CAD build for the part. Positions are in the model's coordinates, mm. Round coordinates to 2 decimals unless told otherwise and drop trailing zeros. Order: outer loops, then holes, each group sorted by start corner. A loop starts at its lowest first (then second) coordinate and runs counter-clockwise, first axis right, second up. Notation, with made-up numbers: (-16.75, -9) - (15.25, -9) arc R5 ccw to (15.25, -3) - close; hole circle Ø9 at (-27.5, 27.25). An arc over 180 degrees is marked (long way). Use one line per item in the form item = value. Start each with the question number.
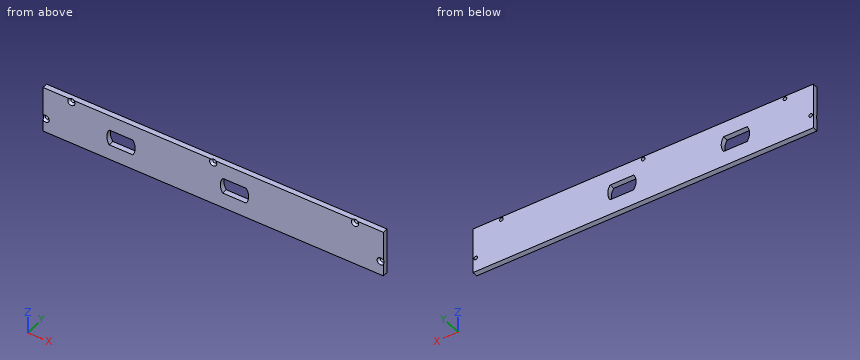
from build123d import *

# Parameters (mm, degrees)
F0_W           = 304.8
F0_H           = 41.275
F1_DEPTH       = 4.7625
F3_D           = 3.2639
F3_DEPTH       = 14.605
F3_CSINK_D     = 6.477
F3_CSINK_ANGLE = 82
F3_TIP         = 0.9805744872
F5_DEPTH       = 25.4


with BuildPart() as f1:
    # F0 (on Front) → F1 (new body)
    with BuildSketch(Plane.XZ):
        with Locations((33.2768968371, 36.1280379981)):
            Rectangle(F0_W, F0_H)
    extrude(amount=F1_DEPTH)

    # F3
    with Locations(Plane.XZ.offset(4.7625)):
        with Locations((-93.7231031629, 54.3842879981), (-116.7418531629, 28.1905379981), (33.2768968371, 54.3842879981), (160.2768968371, 54.3842879981), (183.2956468371, 28.1905379981)):
            CounterSinkHole(F3_D / 2, F3_CSINK_D / 2, depth=F3_DEPTH, counter_sink_angle=F3_CSINK_ANGLE)
            with Locations((0, 0, -(F3_DEPTH + F3_TIP / 2))):  # 118° drill point
                Cone(0, F3_D / 2, F3_TIP, mode=Mode.SUBTRACT)

    # F4 (on face) → F5 (cut)
    with BuildSketch(Plane.XZ.offset(4.7625)):
        with BuildLine():
            Line((-38.6665120517, 43.1130379981), (-59.879694274, 43.1130379981))
            ThreePointArc((-59.879694274, 43.1130379981), (-61.9731031629, 36.1280379981), (-59.879694274, 29.1430379981))
            Line((-59.879694274, 29.1430379981), (-38.6665120517, 29.1430379981))
            ThreePointArc((-38.6665120517, 29.1430379981), (-36.5731031629, 36.1280379981), (-38.6665120517, 43.1130379981))
        make_face()
        with BuildLine():
            ThreePointArc((62.9334879483, 29.1430379981), (65.0268968371, 36.1280379981), (62.9334879483, 43.1130379981))
            Line((62.9334879483, 43.1130379981), (41.720305726, 43.1130379981))
            ThreePointArc((41.720305726, 43.1130379981), (39.6268968371, 36.1280379981), (41.720305726, 29.1430379981))
            Line((41.720305726, 29.1430379981), (62.9334879483, 29.1430379981))
        make_face()
    extrude(amount=-F5_DEPTH, mode=Mode.SUBTRACT)


solid = f1.part
(1) Flat gauge pins, fed straight in: P1, Ø3, axis at x = -93.72, z = 54.38, coming from the +Y side; P2, Ø5, axis at x = 183.3, z = 28.19, coming from the -Y side; P3, Ø4, axis at x = 160.28, z = 54.38, coming from the -Y side. Where does each tip first touch, or does it go through?
(2) Slice it at A-A (z = 40.5). Give the cut face in (x, y), and give its area (3 significant figures).
(3) Wall check: line 1 (X direction, y = -0.85, z = 35.5); line 2 (X direction, y = -1.25, z = 42); line 3 (Z direction, x = 57, y = -1.3). Give the ranges that are in metal, low to high. Write a range as [from, to].
(4) Slice it at B-B (y = -1.7). Give the cut face in (x, z), and give its area (3 significant figures).
Results list:
q1.P1 = through
q1.P2 = -3.92
q1.P3 = -3.34
q2.outline = (-119.12, -4.76) - (-61.2, -4.76) - (-61.2, 0) - (-119.12, 0) - close; (-37.35, -4.76) - (40.4, -4.76) - (40.4, 0) - (-37.35, 0) - close; (64.25, -4.76) - (185.68, -4.76) - (185.68, 0) - (64.25, 0) - close
q2.area = 1,220 mm²
q3.line_1 = [-119.12, -61.96], [-36.59, 39.64], [65.01, 185.68]
q3.line_2 = [-119.12, -60.53], [-38.01, 41.07], [63.59, 185.68]
q3.line_3 = [15.49, 29.14], [43.11, 56.77]
q4.outline = (-119.12, 15.49) - (185.68, 15.49) - (185.68, 56.77) - (-119.12, 56.77) - close; hole circle Ø3.26 at (-116.74, 28.19); hole circle Ø3.26 at (-93.72, 54.38); hole (-59.88, 29.14) - (-38.67, 29.14) arc R12.7 ccw to (-38.67, 43.11) - (-59.88, 43.11) arc R12.7 ccw to start; hole circle Ø3.26 at (33.28, 54.38); hole (41.72, 29.14) - (62.93, 29.14) arc R12.7 ccw to (62.93, 43.11) - (41.72, 43.11) arc R12.7 ccw to start; hole circle Ø3.26 at (160.28, 54.38); hole circle Ø3.26 at (183.3, 28.19)
q4.area = 11,900 mm²
